The listing builds one solid part. Answer for the finished solid, in the listing's coordinates (mm). A direction names the side the tool comes from. Round coordinates to 2 decimals unless told otherwise and drop trailing zeros. Order: outer loops, then holes, each group sorted by start corner. A loop starts at its lowest first (then second) coordinate and runs counter-clockwise, first axis right, second up. Notation, with made-up numbers: M 20.25,79 L 35.25,79 A9 cw 35.25,92 Z; hole C -37.5,58 d11. An arc over 180 degrees is marked long. Write item = value, one per line. Start each with the question number.
(1) A cutting plane is placed at D-D, the plane y = 1.5. Determine the outline of the cut face in (x, z).
(2) Straight lines are drawn through the part: probe 1 along X at (y, z) = (2.25, 32.5); probe 2 along X at (y, z) = (11.75, 21); probe 3 along Y at (x, z) = (-3.05, 29). For each, find the intervals that lie inside material, in ascending order. Write a range as from..to.
(3) For a pull along X with two mould halves and no side action, classify faces 1 (the face through (-0.8, 5, 40)), 2 (the face through (-4.715, 2.597, 39.699)), 3 (the face through (-1, 7, 20)) as released by +X, released by -X, zero draft, split by the parting line, or undercut.
(4) A cutting plane is placed at C-C, the plane x = -3.6. Determine the outline of the cut face in (y, z), and give its area (3 significant figures).
(5) This flat-tipped pin is pushed along its axis until it touches: pin 1 (0.8 mm diameter, centred on x = -2.5, z = 27, fed in from +Y). Where does it stop, or does it pass through?
(6) Which of the six approach directions +Z, -Z, +X, -X, +Y, -Y give full straight-line access (tool end or side, diameter ignored) to faces 4 (the face through (0, 7, 20)), 5 (the face through (-2.5, 1, 19.7))?
(7) A cutting plane is placed at B-B, the plane z = 25.5. Determine the outline of the cut face in (x, y), and give its area (3 significant figures).
from build123d import *

# Parameters (mm, degrees)
F1_DEPTH    = 40
F2_T1_DEPTH = 48.6602540378
F3_R        = 0.99999


# Not quite as in the source:
# - a fillet or chamfer that OpenCascade refuses, or shapes differently, is made with other operations: its cross-section is extruded or revolved along the edge and cut away or added
# - a fillet or chamfer is up to 0.001 mm smaller than in the source, because OpenCascade refuses the exact size


with BuildPart() as f1:
    # F0 (on Top) → F1 (new body)
    with BuildSketch(Plane.XY):
        Polygon((-5, 0), (0, 0), (0, 14), (-1, 14), (-1, 1), (-4, 1), (-4, 7), (-5, 7), align=None)
    extrude(amount=F1_DEPTH)

    # F2: fillet of radius 2 on 2 edges, made by hand

    # F2_s2 → F2_t1 (cut)
    with BuildSketch(Plane.XY.offset(-4.3301270189)):
        with BuildLine():
            ThreePointArc((-4, 7), (-4.7320508076, 6.2679491924), (-5, 5.2679491924))
            Line((-5, 5.2679491924), (-5, 7))
            Line((-5, 7), (-4, 7))
        make_face()
        with BuildLine():
            ThreePointArc((0, 14), (-0.7320508076, 13.2679491924), (-1, 12.2679491924))
            Line((-1, 12.2679491924), (-1, 14))
            Line((-1, 14), (0, 14))
        make_face()
    extrude(amount=F2_T1_DEPTH, mode=Mode.SUBTRACT)

    # F3 (radius 1 in the source; OpenCascade refuses exactly that, so slightly less here)
    f3_edges = [f1.edges().sort_by_distance(p)[0] for p in [
        (-5, 2.633975, 40),
        (-5, 2.633975, 0),
        (-5, 0, 20),
        (0, 0, 20),
        (-4, 1, 20),
        (-1, 1, 20),
        (-4.732051, 6.267949, 0),
        (-4.732051, 6.267949, 40),
    ]]
    fillet(f3_edges, radius=F3_R)


solid = f1.part
Reported:
q1.outline = M -5,1 A1 ccw -4,0 L -3.87,0 L -3.87,40 L -4,40 A1 ccw -5,39 Z; M -1.13,0 L 0,0 L 0,40 L -1.13,40 Z
q2.probe_1 = -5..-4, -1..0
q2.probe_2 = -1..0
q2.probe_3 = 0..1
q3.face_1 = zero draft
q3.face_2 = released by -X
q3.face_3 = undercut
q4.outline = M 0,0 L 1.2,0 L 1.2,40 L 0,40 Z
q4.area = 48.0 mm²
q5.pin_1 = 1
q6.face_4 = +Z, -Z, +X, +Y, -Y
q6.face_5 = +Z, -Z, +Y
q7.outline = M -5,1 A1 ccw -4,0 L -1,0 A1 ccw 0,1 L 0,14 A2 ccw -1,12.27 L -1,2 A1 cw -2,1 L -3,1 A1 cw -4,2 L -4,7 A2 ccw -5,5.27 Z
q7.area = 23.0 mm²
